Input: dimensioned drawing with shaded views. Units: mm. Origin: part minimum x, y, z. A direction names the side the tool comes from. Give positions to 0.01 mm unless a question says otherwise; leave off trailing zeros. Loops run counter-clockwise (first coordinate to the right, second up) from the corner with the lowest first, then second, coordinate; pieces in that order, holes last. Notation, with made-up numbers: M -36.75,63 L -0.75,63 A15 ccw -0.75,80 Z; hole C 45,2 d11. An arc over 180 degrees is marked long. One line per question, with ' | ' between items. Start each with the question number.
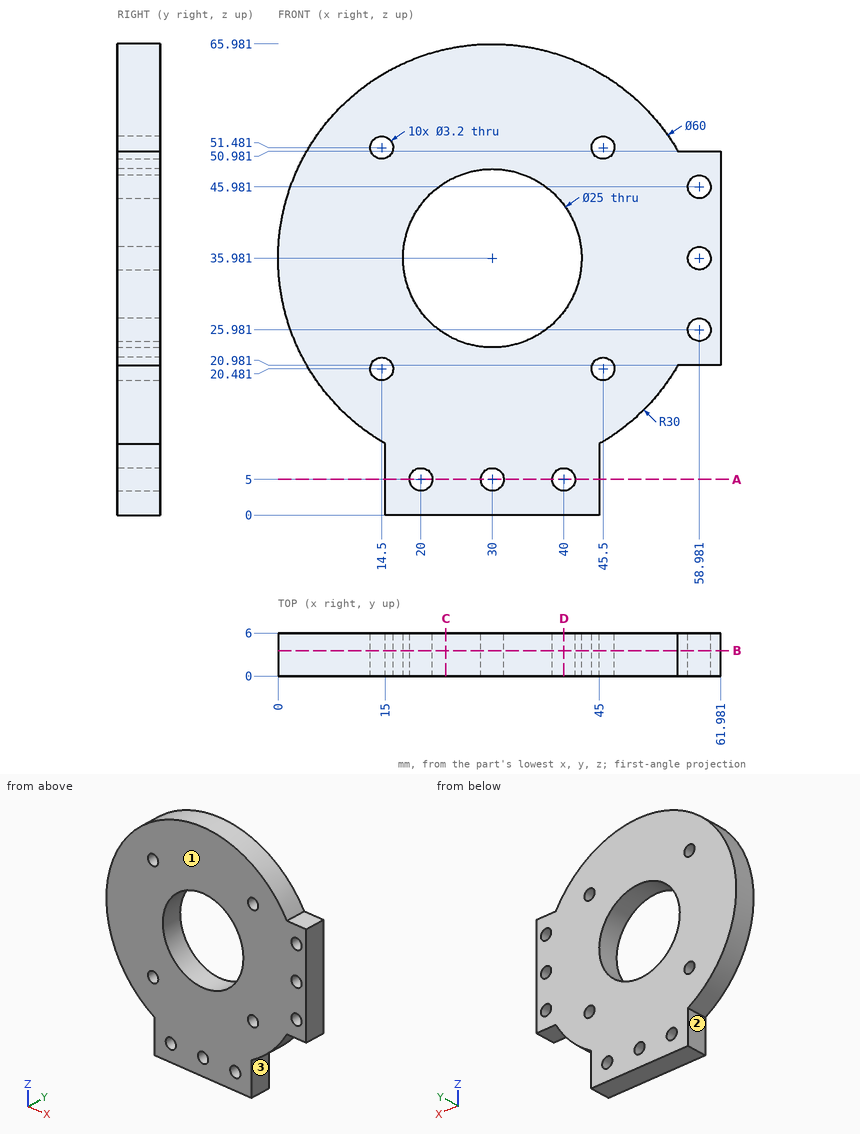
Q1. Material intervals for L1, parallel to X at y = 0.9, z = 38; L2, parallel to X at y = 2.5, z = 20 (1 decimal); L3, parallel to X at y = 2.15, z = 32.5 (1 decimal), sorted ascending.
Q2. Set-up query: the marked faces 1, 2 and 3. Return all of +Z, -Z, +X, -X, +Y, -Y with unobstructed straight access to the full face (end or side cutting, diameter ignored); none if empty.
Q3. Section A-A, the plane z = 5. Output: boundary loops of the cut face in (x, y).
Q4. Section B-B, the plane y = 3.55. Count the separate pieces of the cut face and the enclosed holes in it, plus the area to 3 significant figures.
Q5. Section C-C, the plane x = 23.5. Output: boundary loops of the cut face in (y, z).
Q6. Contact query for flat-ended pins moving along their axis: pin 1 (3 mm diameter, centred on x = 58.98, z = 35.98, fed in from +Y); pin 2 (1.5 mm diameter, centred on x = 47, y = 1, fed in from -Z); pin 3 (3 mm diameter, centred on y = 2.5, z = 19.5, fed in from -X); pin 4 (3 mm diameter, centred on x = 60.5, y = 3, fed in from +Z). Output: stop coordinate, or through.
Q7. Section D-D, the plane x = 40. Output: boundary loops of the cut face in (y, z) (1 decimal), plus the area to 3 significant figures.
Model answer:
1) L1: x = 0.07 to 17.66, 42.34 to 61.98 | L2: x = 4.6 to 13, 16 to 44, 47 to 55.4 | L3: x = 0.2 to 18, 42 to 62
2) face 1: +Z, -Z, +X, -X, -Y | face 2: -Z, -X, +Y, -Y | face 3: -Z, +X, +Y, -Y
3) outline: M 15,0 L 18.4,0 L 18.4,6 L 15,6 Z; M 21.6,0 L 28.4,0 L 28.4,6 L 21.6,6 Z; M 31.6,0 L 38.4,0 L 38.4,6 L 31.6,6 Z; M 41.6,0 L 45,0 L 45,6 L 41.6,6 Z
4) separate pieces: 1 | enclosed holes: 11 | area: 2,570 mm^2
5) outline: M 0,0 L 6,0 L 6,25.3 L 0,25.3 Z; M 0,46.66 L 6,46.66 L 6,65.27 L 0,65.27 Z
6) pin 1: passes through | pin 2: stops at z = 10.76 | pin 3: stops at x = 4.01 | pin 4: stops at z = 50.98
7) outline: M 0,0 L 6,0 L 6,3.4 L 0,3.4 Z; M 0,6.6 L 6,6.6 L 6,28.5 L 0,28.5 Z; M 0,43.5 L 6,43.5 L 6,64.3 L 0,64.3 Z | area: 276 mm^2
